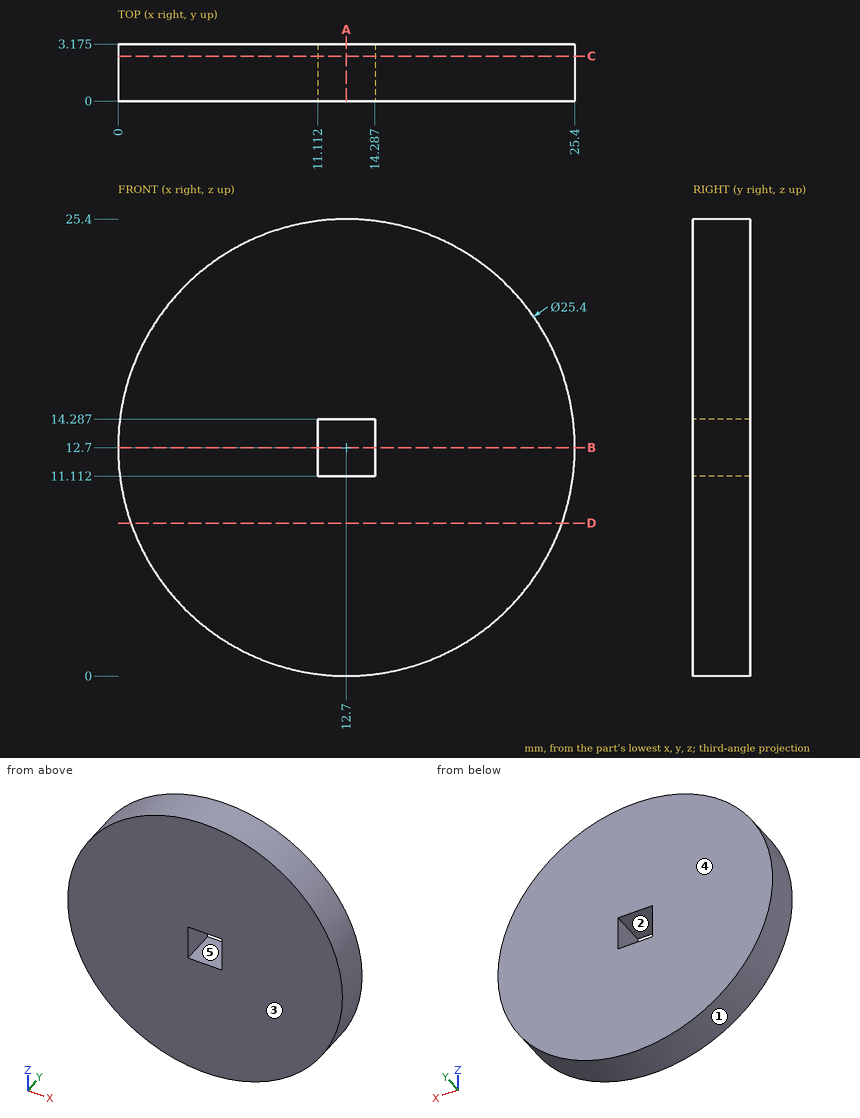
Check sheet for the drawn part. Datum: minimum x, y, z corner. Units: mm. A direction names the side the tool comes from. Give positions to 0.01 mm unless a question says otherwise; leave off trailing zeros. Order: outer loops, then holes, each group sorted by start corner. A loop starts at its lowest first (then second) coordinate and runs counter-clockwise, first axis right, second up. Notation, with made-up numbers: (-32.75, -24.5) - (-18.75, -24.5) arc R27 cw to (-18.75, 12.5) - close; hole circle Ø6 at (-23, 80.25). An arc over 180 degrees is marked (long way). Write item = value, one per line. Start each with the question number.
1) Access from +Z, -Z, +X, -X, +Y, -Y to the whole of each face (thin tool, end or side, straight path). Record for the marked faces 4 and 5.
2) Gauge pin test, flat end, axial feed: pin 1 Ø5 at (x, z) = (14.5, 21) entering from -Y. Record the tip position at first contact, or that the pin passes through.
3) Section check B-B (z = 12.7). Enter the section's corners in (x, y) (1 decimal).
4) Section check D-D (z = 8.5). Enter the section's corners in (x, y) (1 decimal).
5) Section check A-A (x = 12.7). Enter the section's corners in (y, z) (1 decimal).
6) Section check C-C (y = 2.5). Enter the section's corners in (x, z).
7) Scan lines: L1, parallel to X at y = 0.7, z = 12.75; L2, parallel to X at y = 0.7, z = 20.75 (1 decimal); L3, parallel to Z at x = 1.75, y = 1.4 (1 decimal). Record each from-to range of solid material in increasing order.
8) Draft check along Z on the marked faces 1, 2 and 3. Enter one of: released by +Z, released by -Z, zero draft, split by the parting line, or undercut.
Geometry check:
q1.face_4 = +Z, -Z, +X, -X, +Y
q1.face_5 = +Y, -Y
q2.pin_1 = 0
q3.outline = (0, 0) - (11.1, 0) - (11.1, 3.2) - (0, 3.2) - close; (14.3, 0) - (25.4, 0) - (25.4, 3.2) - (14.3, 3.2) - close
q4.outline = (0.7, 0) - (24.7, 0) - (24.7, 3.2) - (0.7, 3.2) - close
q5.outline = (0, 0) - (3.2, 0) - (3.2, 11.1) - (0, 11.1) - close; (0, 14.3) - (3.2, 14.3) - (3.2, 25.4) - (0, 25.4) - close
q6.outline = circle Ø25.4 at (12.7, 12.7); hole (11.11, 11.11) - (14.29, 11.11) - (14.29, 14.29) - (11.11, 14.29) - close
q7.L1 = 0 to 11.11, 14.29 to 25.4
q7.L2 = 2.9 to 22.5
q7.L3 = 6.3 to 19.1
q8.face_1 = split by the parting line
q8.face_2 = undercut
q8.face_3 = zero draft
